Read the model definition and answer for the solid it produces. Units are mm, in the model's axes. A direction names the side the tool comes from. Coordinates: 2 decimals unless noted, no trailing zeros. Loops run counter-clockwise (first coordinate to the right, second up) from the corner with the lowest first, then second, coordinate; pieces in that order, holes last.
from build123d import *

# Parameters (mm, degrees)
F0_W     = 50.8
F0_H     = 69.85
F1_DEPTH = 12.7
F2_R     = 6.35
F3_DEPTH = 31.75
F4_DEPTH = 12.7


with BuildPart() as f1:
    # F0 (on Front) → F1 (new body)
    with BuildSketch(Plane.XZ):
        with Locations((-18.859848, 4.442824)):
            Rectangle(F0_W, F0_H)
    extrude(amount=F1_DEPTH)

    # F2 (on face) → F3 (cut)
    with BuildSketch(Plane.XZ.offset(12.7)):
        with BuildLine():
            Line((-31.559848, -24.132176), (-31.559848, 26.667824))
            ThreePointArc((-31.559848, 26.667824), (-27.840104, 35.64808), (-18.859848, 39.367824))
            Line((-18.859848, 39.367824), (-44.259848, 39.367824))
            Line((-44.259848, 39.367824), (-44.259848, -30.482176))
            Line((-44.259848, -30.482176), (-37.909848, -30.482176))
            ThreePointArc((-37.909848, -30.482176), (-33.41972, -28.622304), (-31.559848, -24.132176))
        make_face()
        with Locations((-18.859848, 26.667824)):
            Circle(F2_R)
        with BuildLine():
            ThreePointArc((-18.859848, 39.367824), (-9.879591, 35.64808), (-6.159848, 26.667824))
            Line((-6.159848, 26.667824), (-6.159848, -24.132176))
            ThreePointArc((-6.159848, -24.132176), (-4.299976, -28.622304), (0.190152, -30.482176))
            Line((0.190152, -30.482176), (6.540152, -30.482176))
            Line((6.540152, -30.482176), (6.540152, 39.367824))
            Line((6.540152, 39.367824), (-18.859848, 39.367824))
        make_face()
    extrude(amount=-F3_DEPTH, mode=Mode.SUBTRACT)

    # F2 (on face) → F4 (join)
    with BuildSketch(Plane.XZ.offset(12.7)):
        with BuildLine():
            ThreePointArc((-31.559848, 26.667824), (-18.859848, 13.967824), (-6.159848, 26.667824))
            ThreePointArc((-6.159848, 26.667824), (-18.859848, 39.367824), (-31.559848, 26.667824))
        make_face()
        with Locations((-18.859848, 26.667824)):
            Circle(F2_R, mode=Mode.SUBTRACT)
    extrude(amount=F4_DEPTH)


solid = f1.part
Item 1: A cutting plane is placed at C-C on x = -33. Determine the outline of the cut face in (y, z).
Numbers:
outline: (-12.7, -30.48) - (0, -30.48) - (0, -28.16) - (-12.7, -28.16) - close
Item 2: Which of the six approach directions +Z, -Z, +X, -X, +Y, -Y give full straight-line access (tool end or side, diameter ignored) to faces 1 (the face through (-6.16, -6, 2)), 2 (the face through (-31.56, -6, 1)), 3 (the face through (-19, -6, -30.482))?
Numbers:
face 1: +Z, +X, +Y, -Y
face 2: +Z, -X, +Y, -Y
face 3: -Z, +X, -X, +Y, -Y
Item 3: A cutting plane is placed at A-A on y = -9. Determine the outline of the cut face in (x, z), then the cut area to 3 significant figures.
Numbers:
outline: (-37.91, -30.48) - (0.19, -30.48) arc R6.35 cw to (-6.16, -24.13) - (-6.16, 26.67) arc R12.7 ccw to (-18.86, 39.37) arc R12.7 ccw to (-31.56, 26.67) - (-31.56, -24.13) arc R6.35 cw to start; hole circle Ø12.7 at (-18.86, 26.67)
area: 1,600 mm2
Item 4: A cutting plane is placed at D-D on y = -15.25. Determine the outline of the cut face in (x, z), then the cut area to 3 significant figures.
Numbers:
outline: circle Ø25.4 at (-18.86, 26.67); hole circle Ø12.7 at (-18.86, 26.67)
area: 380 mm2
Item 5: A cutting plane is placed at B-B on z = 35.5. Determine the outline of the cut face in (x, y), then the cut area to 3 significant figures.
Numbers:
outline: (-27.99, -25.4) - (-9.73, -25.4) - (-9.73, 0) - (-27.99, 0) - close
area: 464 mm2
Item 6: Given pin 1 (5 mm diameter, centred on y = -14.5, z = -20.5, fed in from +X); pin 2 (19 mm diameter, centred on x = -14.5, z = -3.5, fed in from -Y); pin 3 (4 mm diameter, centred on y = -6, z = 2.5, fed in from -X); pin 4 (10 mm diameter, centred on x = -18.86, z = 26.67, fed in from +Y), each flat-ended and moving along its own axis, determine where each tip first touches the part or whether it passes through.
Numbers:
pin 1: stops at x = -6.16
pin 2: stops at y = -12.7
pin 3: stops at x = -31.56
pin 4: passes through
Item 7: Find the intervals of material crossed by line 1 along Z through (x, y) = (-18.5, -17); line 2 along Y through (x, z) = (-15, -20.5); line 3 along X through (y, z) = (-1.25, -16), in increasing order.
Numbers:
line 1: z = 13.97 to 20.33, 33.01 to 39.36
line 2: y = -12.7 to 0
line 3: x = -31.56 to -6.16
